CAD build for the part. Positions are in the model's coordinates, mm. A direction names the side the tool comes from. Round coordinates to 2 decimals unless told otherwise and drop trailing zeros. Loops run counter-clockwise (first coordinate to the right, second up) from the corner with the lowest first, then second, coordinate; pieces in that order, holes last.
```python
from build123d import *

# Parameters (mm, degrees)
SKETCH1_R                    = 3.25
BASE_FLANGE1_DEPTH           = 3.175
EDGE_FLANGE1_STRIP_W         = 15.24
EDGE_FLANGE1_STRIP_H         = 3.175
EDGE_FLANGE1_STRIP_CUT_DEPTH = 18
EDGE_FLANGE1_DEPTH           = 18
EDGE_FLANGE2_STRIP_W         = 15.24
EDGE_FLANGE2_STRIP_H         = 3.175
EDGE_FLANGE2_STRIP_CUT_DEPTH = 18
EDGE_FLANGE2_DEPTH           = 18
SKETCH12_R                   = 4.125
BOSS_EXTRUDE1_DEPTH          = 3.175


# Sheet-metal steps are written as plain solids
with BuildPart() as part:
    # Sketch1 → Base-Flange1 (new body)
    with BuildSketch(Plane(origin=(0, 0, 0), x_dir=(1, 0, 0), z_dir=(0, 1, 0))):
        with BuildLine():
            Line((-7, 10), (-7, 0))
            ThreePointArc((-7, 0), (-4.949747468, -4.949747468), (0, -7))
            Line((0, -7), (4, -7))
            ThreePointArc((4, -7), (8.949747468, -4.949747468), (11, 0))
            Line((11, 0), (11, 10))
            Line((11, 10), (-7, 10))
        make_face()
        with Locations(Location((0, 0, 0), (0, 0, 270))):
            Circle(SKETCH1_R, mode=Mode.SUBTRACT)
    extrude(amount=-BASE_FLANGE1_DEPTH)

    # Edge-Flange1 strip (across the edge) → Edge-Flange1 strip cut (cut)
    with BuildSketch(Plane(origin=(11, 0, -10), x_dir=(0, 0, 1), z_dir=(-1, 0, 0))):
        with Locations((-6.35, -1.5875)):
            Rectangle(EDGE_FLANGE1_STRIP_W, EDGE_FLANGE1_STRIP_H)
    extrude(amount=EDGE_FLANGE1_STRIP_CUT_DEPTH, mode=Mode.SUBTRACT)

    # Edge-Flange1 section (across the edge) → Edge-Flange1 (add)
    with BuildSketch(Plane(origin=(11, 0, -10), x_dir=(0, 0, 1), z_dir=(-1, 0, 0))):
        with BuildLine():
            Line((-3.175, 1.27), (-3.175, 45.0625))
            Line((-3.175, 45.0625), (0, 45.0625))
            Line((0, 45.0625), (0, 1.27))
            ThreePointArc((0, 1.27), (0.371974388, 0.371974388), (1.27, 0))
            Line((1.27, 0), (1.27, -3.175))
            ThreePointArc((1.27, -3.175), (-1.873089642, -1.873089642), (-3.175, 1.27))
        make_face()
    extrude(amount=EDGE_FLANGE1_DEPTH)

    # Edge-Flange2 strip (across the edge) → Edge-Flange2 strip cut (cut)
    with BuildSketch(Plane(origin=(-7, 45.0625, -13.175), x_dir=(0, -1, 0), z_dir=(1, 0, 0))):
        with Locations((-6.35, -1.5875)):
            Rectangle(EDGE_FLANGE2_STRIP_W, EDGE_FLANGE2_STRIP_H)
    extrude(amount=EDGE_FLANGE2_STRIP_CUT_DEPTH, mode=Mode.SUBTRACT)

    # Edge-Flange2 section (across the edge) → Edge-Flange2 (add)
    with BuildSketch(Plane(origin=(-7, 45.0625, -13.175), x_dir=(0, -1, 0), z_dir=(1, 0, 0))):
        with BuildLine():
            Line((-3.175, 1.27), (-3.175, 3))
            Line((-3.175, 3), (0, 3))
            Line((0, 3), (0, 1.27))
            ThreePointArc((0, 1.27), (0.371974388, 0.371974388), (1.27, 0))
            Line((1.27, 0), (1.27, -3.175))
            ThreePointArc((1.27, -3.175), (-1.873089642, -1.873089642), (-3.175, 1.27))
        make_face()
    extrude(amount=EDGE_FLANGE2_DEPTH)

    # Sketch12 → Boss-Extrude1 (add)
    with BuildSketch(Plane(origin=(0, 48.2375, 0), x_dir=(1, 0, 0), z_dir=(0, 1, 0))):
        with BuildLine():
            Line((11, 16.175), (-7, 16.175))
            ThreePointArc((-7, 16.175), (-4.820309554, 27.006048634), (1.379401037, 36.150787753))
            Line((1.379401037, 36.150787753), (27.144104233, 61.457369654))
            ThreePointArc((27.144104233, 61.457369654), (32.821748623, 63.749679884), (38.457357581, 61.355887143))
            Line((38.457357581, 61.355887143), (39.858828935, 59.92904516))
            ThreePointArc((39.858828935, 59.92904516), (42.151139165, 54.251400771), (39.757346424, 48.615791813))
            Line((39.757346424, 48.615791813), (13.992643228, 23.309209912))
            ThreePointArc((13.992643228, 23.309209912), (11.778460873, 20.043231655), (11, 16.175))
        make_face()
        with Locations(Location((32.749989651, 55.750001725, 0), (0, 0, 270))):
            Circle(SKETCH12_R, mode=Mode.SUBTRACT)
    extrude(amount=-BOSS_EXTRUDE1_DEPTH)


solid = part.part
```
Item 1: Cut at C-C, the plane z = -35. Give the cut face in (x, y).
Answers follow:
outline: (0.27, 45.06) - (25.9, 45.06) - (25.9, 48.24) - (0.27, 48.24) - close
Item 2: Two-plate mould, pull along Z, no slides. Class faces 4 (the flat face through (2, -3.175, -3)), 5 (the cylindrical face through (32.73, 46.67, -63.75)), 6 (the cylindrical face through (-1.978, -1.565, -2.579)): released by +Z, released by -Z, zero draft, split by the parting line, or undercut.
Answers follow:
face 4: zero draft
face 5: released by -Z
face 6: undercut
Item 3: 3-axis set-ups, long thin cutter, end or side, ignore diameter. For faces 1 (the cylindrical face through (-4.88, 46.67, -26.86)), 2 (the flat face through (2, 0, -3)), 3 (the flat face through (2, 22, -13.175)): which of +Z, -Z, +X, -X, +Y, -Y reach the whole face in a straight line?
Answers follow:
face 1: -Z, -X, +Y, -Y
face 2: +Z, +X, -X, +Y
face 3: -Z, +X, -X, -Y
Item 4: Probe line 1 (X direction, y = -0.65, z = 0); line 2 (Z direction, x = 7.5, y = 37) (3 decimals); line 3 (Y direction, x = 23.5, z = -50.5). List the from-to ranges inside material, lowest first.
Answers follow:
line 1: x = -7 to -3.25, 3.25 to 11
line 2: z = -13.175 to -10
line 3: y = 45.06 to 48.24
Item 5: Cut at B-B, the plane y = 13.5. Give the cut face in (x, z) (3 decimals), plus the area to 4 significant figures.
Answers follow:
outline: (-7, -13.175) - (11, -13.175) - (11, -10) - (-7, -10) - close
area: 57.15 mm2
Item 6: Flat gauge pins, fed straight in: P1, Ø3, axis at x = 11.5, y = 42.5, coming from the +Z side; P2, Ø5.5, axis at x = 5.5, y = 18, coming from the -Z side (3 decimals); P3, Ø8, axis at y = 19, z = -4.5, coming from the +X side; P4, Ø14.5, axis at x = 20.5, z = -31, coming from the -Y side. Where does each tip first touch, or does it go through?
Answers follow:
P1: stops at z = -10
P2: stops at z = -13.175
P3: passes through
P4: stops at y = 45.06
Item 7: Cut at A-A, the plane x = 6. Give the cut face in (y, z) (1 decimal).
Answers follow:
outline: (-3.2, -8.7) arc R4.4 ccw to (1.3, -13.2) - (43.8, -13.2) arc R1.3 cw to (45.1, -14.4) - (45.1, -40.7) - (48.2, -40.7) - (48.2, -14.4) arc R4.4 ccw to (43.8, -10) - (1.3, -10) arc R1.3 cw to (0, -8.7) - (0, 6.7) - (-3.2, 6.7) - close
